Verification items for the finished model (mm, model axes). A direction names the side the tool comes from. Coordinates: 2 decimals unless noted, no trailing zeros. Write each loop counter-clockwise with the first axis right and the second up, starting at its lowest first coordinate (ties: lowest second). Pieces come first, ordered by that corner, then holes. Notation, with made-up numbers: (15.5, -0.75) -> (51.5, -0.75) arc R26 ccw to (51.5, 30.25) -> close; hole circle Ø9 at (86.5, 87). An arc over 180 degrees is marked (long way). Write item = value, one per line. Start each with the question number.
(1) Set-up check for faces 4 (the face through (13.9, 2.22, -14.43)), 5 (the face through (-2.863, 2.218, -4.454)): record each of +Z, -Z, +X, -X, +Y, -Y from which the full face is reachable in a straight line by a thin tool's end or side.
(2) Section check B-B (y = 3.65). Record the cut outline in (x, z).
(3) Section check A-A (x = 0). Record the cut outline in (y, z), plus the area to 3 significant figures.
(4) Mould release check, pull along X, two halves, no side actions. Record for faces 1 (the face through (-13.9, 2.22, 11.43)), 2 (the face through (13.93, 2.22, 11.4)), 3 (the face through (-4, 2, 8)): released by +X, released by -X, zero draft, split by the parting line, or undercut.
(5) Section check D-D (z = -1.5). Record the cut outline in (x, y).
(6) Material ranges on probe 1 along X at (y, z) = (2.75, -10); probe 2 along Z at (x, y) = (-10, 2.7); probe 3 along X at (y, z) = (3.8, -0.25), recorded low to high. Write a range as [from, to].
(7) Section check C-C (z = -5). Record the cut outline in (x, y), plus the area to 3 significant figures.
```python
from build123d import *

# Parameters (mm, degrees)
SKETCH3_R           = 1.55
BOSS_EXTRUDE1_DEPTH = 4.5


with BuildPart() as part:
    # Sketch3 → Boss-Extrude1 (new body)
    with BuildSketch(Plane(origin=(0, 0, 0), x_dir=(1, 0, 0), z_dir=(0, 1, 0))):
        with BuildLine():
            Line((-14.5, -10), (-14.5, 13))
            ThreePointArc((-14.5, 13), (-13.914213562, 14.414213562), (-12.5, 15))
            Line((-12.5, 15), (12.5, 15))
            ThreePointArc((12.5, 15), (13.914213562, 14.414213562), (14.5, 13))
            Line((14.5, 13), (14.5, -10))
            ThreePointArc((14.5, -10), (13.914213562, -11.414213562), (12.5, -12))
            Line((12.5, -12), (-12.5, -12))
            ThreePointArc((-12.5, -12), (-13.914213562, -11.414213562), (-14.5, -10))
        make_face()
        with Locations(Location((10, 10, 0), (0, 0, 270))):
            Circle(SKETCH3_R, mode=Mode.SUBTRACT)
        with Locations(Location((11, -8, 0), (0, 0, 270))):
            Circle(SKETCH3_R, mode=Mode.SUBTRACT)
        with Locations(Location((-11, -8, 0), (0, 0, 90))):
            Circle(SKETCH3_R, mode=Mode.SUBTRACT)
        with Locations(Location((-10, 10, 0), (0, 0, 90))):
            Circle(SKETCH3_R, mode=Mode.SUBTRACT)
        with BuildLine():
            Line((3.094753625, -4.905354218), (3.094753625, -8))
            Line((3.094753625, -8), (5.123475383, -8))
            ThreePointArc((5.123475383, -8), (8.227241336, -4.75), (9.489940922, -0.437059837))
            Line((9.489940922, -0.437059837), (4.366465539, 8.437059837))
            ThreePointArc((4.366465539, 8.437059837), (0, 9.5), (-4.366465539, 8.437059837))
            Line((-4.366465539, 8.437059837), (-9.489940922, -0.437059837))
            ThreePointArc((-9.489940922, -0.437059837), (-8.227241336, -4.75), (-5.123475383, -8))
            Line((-5.123475383, -8), (-3.094753625, -8))
            Line((-3.094753625, -8), (-3.094753625, -4.905354218))
            ThreePointArc((-3.094753625, -4.905354218), (-5.776273327, -0.524086301), (-3.927083333, 4.268256845))
            ThreePointArc((-3.927083333, 4.268256845), (-2.848181218, 4.4480697), (-2.25, 3.532350492))
            Line((-2.25, 3.532350492), (-2.25, 0))
            ThreePointArc((-2.25, 0), (0, -2.25), (2.25, 0))
            Line((2.25, 0), (2.25, 3.532350492))
            ThreePointArc((2.25, 3.532350492), (2.848181218, 4.4480697), (3.927083333, 4.268256845))
            ThreePointArc((3.927083333, 4.268256845), (5.776273327, -0.524086301), (3.094753625, -4.905354218))
        make_face(mode=Mode.SUBTRACT)
    extrude(amount=BOSS_EXTRUDE1_DEPTH)


solid = part.part
```
Response:
q1.face_4 = -Z, +X, +Y, -Y
q1.face_5 = +Y, -Y
q2.outline = (-14.5, -13) arc R2 ccw to (-12.5, -15) -> (12.5, -15) arc R2 ccw to (14.5, -13) -> (14.5, 10) arc R2 ccw to (12.5, 12) -> (-12.5, 12) arc R2 ccw to (-14.5, 10) -> close; hole circle Ø3.1 at (-11, 8); hole circle Ø3.1 at (-10, -10); hole (-9.49, 0.44) -> (-4.37, -8.44) arc R9.5 ccw to (4.37, -8.44) -> (9.49, 0.44) arc R9.5 ccw to (5.12, 8) -> (3.09, 8) -> (3.09, 4.91) arc R5.8 cw to (3.93, -4.27) arc R1 cw to (2.25, -3.53) -> (2.25, 0) arc R2.25 ccw to (-2.25, 0) -> (-2.25, -3.53) arc R1 cw to (-3.93, -4.27) arc R5.8 cw to (-3.09, 4.91) -> (-3.09, 8) -> (-5.12, 8) arc R9.5 ccw to start; hole circle Ø3.1 at (10, -10); hole circle Ø3.1 at (11, 8)
q3.outline = (0, -15) -> (4.5, -15) -> (4.5, -9.5) -> (0, -9.5) -> close; (0, 2.25) -> (4.5, 2.25) -> (4.5, 12) -> (0, 12) -> close
q3.area = 68.6 mm2
q4.face_1 = released by -X
q4.face_2 = released by +X
q4.face_3 = undercut
q5.outline = (-14.5, 0) -> (-8.37, 0) -> (-8.37, 4.5) -> (-14.5, 4.5) -> close; (-5.6, 0) -> (-2.25, 0) -> (-2.25, 4.5) -> (-5.6, 4.5) -> close; (2.25, 0) -> (5.6, 0) -> (5.6, 4.5) -> (2.25, 4.5) -> close; (8.37, 0) -> (14.5, 0) -> (14.5, 4.5) -> (8.37, 4.5) -> close
q6.probe_1 = [-14.5, -11.55], [-8.45, 8.45], [11.55, 14.5]
q6.probe_2 = [-15, -11.55], [-8.45, 6.82], [9.18, 12]
q6.probe_3 = [-14.5, -9.09], [-5.79, -2.25], [2.25, 5.79], [9.09, 14.5]
q7.outline = (-14.5, 0) -> (-6.35, 0) -> (-6.35, 4.5) -> (-14.5, 4.5) -> close; (6.35, 0) -> (14.5, 0) -> (14.5, 4.5) -> (6.35, 4.5) -> close
q7.area = 73.3 mm2
